from build123d import *

# Parameters (mm, degrees)
SKETCH1_W           = 5
SKETCH1_H           = 157
BOSS_EXTRUDE1_DEPTH = 30.4
SKETCH2_W           = 5
SKETCH2_H           = 2.9
BOSS_EXTRUDE2_DEPTH = 6
SKETCH3_R           = 1.05
CUT_EXTRUDE1_DEPTH  = 161.02862244
SKETCH4_R           = 2
CUT_EXTRUDE2_DEPTH  = 1.4
FILLET1_R           = 4
FILLET2_R           = 2.5


with BuildPart() as part:
    # Sketch1 → Boss-Extrude1 (new body)
    with BuildSketch(Plane(origin=(0, 0, 0), x_dir=(1, 0, 0), z_dir=(0, 1, 0))):
        with Locations((-2.5, 78.5)):
            Rectangle(SKETCH1_W, SKETCH1_H)
    extrude(amount=BOSS_EXTRUDE1_DEPTH)

    # Sketch2 → Boss-Extrude2 (add)
    with BuildSketch(Plane(origin=(0, 0, 0), x_dir=(0, 0, -1), z_dir=(1, 0, 0))):
        with Locations((2.5, 28.95)):
            Rectangle(SKETCH2_W, SKETCH2_H)
        with Locations((41.5, 28.95)):
            Rectangle(SKETCH2_W, SKETCH2_H)
        with Locations((41.5, 1.45)):
            Rectangle(SKETCH2_W, SKETCH2_H)
        with Locations((2.5, 1.45)):
            Rectangle(SKETCH2_W, SKETCH2_H)
    extrude(amount=BOSS_EXTRUDE2_DEPTH)

    # Sketch3 → Cut-Extrude1 (cut, through all)
    with BuildSketch(Plane(origin=(0, 30.4, 0), x_dir=(1, 0, 0), z_dir=(0, 1, 0))):
        with Locations(Location((3.5, 41.5, 0), (0, 0, 270))):
            Circle(SKETCH3_R)
        with Locations(Location((3.5, 2.5, 0), (0, 0, 270))):
            Circle(SKETCH3_R)
    extrude(amount=-CUT_EXTRUDE1_DEPTH, mode=Mode.SUBTRACT)

    # Sketch4 → Cut-Extrude2 (cut)
    with BuildSketch(Plane(origin=(0, 30.4, 0), x_dir=(1, 0, 0), z_dir=(0, 1, 0))):
        with Locations(Location((3.5, 41.5, 0), (0, 0, 270))):
            Circle(SKETCH4_R)
        with Locations(Location((3.5, 2.5, 0), (0, 0, 270))):
            Circle(SKETCH4_R)
    cut_extrude2 = extrude(amount=-CUT_EXTRUDE2_DEPTH, mode=Mode.SUBTRACT)

    # Mirror2: Cut-Extrude2 across plane
    add(cut_extrude2.mirror(Plane.ZX.offset(15.2)), mode=Mode.SUBTRACT)

    # Fillet1
    fillet1_edges = [part.edges().sort_by_distance(p)[0] for p in [
        (-2.5, 0, -157),
        (-5, 15.2, 0),
        (-2.5, 30.4, -157),
    ]]
    fillet(fillet1_edges, radius=FILLET1_R)

    # Fillet2
    fillet2_edges = [part.edges().sort_by_distance(p)[0] for p in [
        (6, 1.45, -5),
        (6, 1.45, 0),
        (6, 1.45, -44),
        (6, 1.45, -39),
        (6, 28.95, -44),
        (6, 28.95, -39),
        (6, 28.95, -5),
        (6, 28.95, 0),
    ]]
    fillet(fillet2_edges, radius=FILLET2_R - 0.0001)  # a hair under: the kernel refuses the full size


solid = part.part
The listing builds one solid part. Answer for the finished solid, in the listing's coordinates (mm). A direction names the side the tool comes from. Give positions to 0.01 mm unless a question says otherwise; leave off trailing zeros. Write each loop counter-clockwise with the first axis right and the second up, starting at its lowest first coordinate (ties: lowest second). Pieces come first, ordered by that corner, then holes.
Item 1: Section B-B, the plane z = -104 is taken. Write down the section's boundary in (x, y).
Item 2: Flat-ended cylindrical pins translate along their axes: P1, Ø1.2, axis at x = 3.5, z = -2, coming from the -Y side; P2, Ø5.5, axis at x = 3.5, z = -40.5, coming from the -Y side; P3, Ø3.5, axis at x = 3.5, z = -41.5, coming from the +Y side; P4, Ø1.3, axis at x = 3.5, z = -2.5, coming from the +Y side. Find the tip coordinate at first contact, or state that the pin passes through.
Item 3: Determine the mould class of faces 1 (the flat face through (2, 2.9, -41)), 2 (the cylindrical face through (5.248, 1.47, -0.713)), 3 (the flat face through (2.6, 29, -40.6)) for opening direction Y: released by +Y, released by -Y, zero draft, split by the parting line, or undercut.
Item 4: Which of the six approach directions +Z, -Z, +X, -X, +Y, -Y give full straight-line access (tool end or side, diameter ignored) to faces 4 (the flat face through (2.6, 1.4, -40.6)), 5 (the flat face through (2, 2.9, -2)), 6 (the flat face through (2, 1, -39))?
Item 5: Section A-A, the plane y = 20.5 is taken. Write down the section's boundary in (x, z), plus the area to 3 significant figures.
Item 6: Find the intervals of material crossed by line 1 along X through (y, z) = (11.5, -78.5); line 2 along X through (y, z) = (2, -2); line 3 along X through (y, z) = (29.5, -2.5), in increasing order.
Completed:
1. outline: (-5, 0) - (0, 0) - (0, 30.4) - (-5, 30.4) - close
2. P1: stops at y = 1.4
2. P2: stops at y = 0
2. P3: stops at y = 29
2. P4: passes through
3. face 1: undercut
3. face 2: zero draft
3. face 3: released by +Y
4. face 4: -Y
4. face 5: +Z, -Z, +X
4. face 6: +X, +Y, -Y
5. outline: (-5, -157) - (0, -157) - (0, 0) - (-1, 0) arc R4 ccw to (-5, -4) - close
5. area: 782 mm2
6. line 1: x = -5 to 0
6. line 2: x = -4.46 to 2.58, 4.42 to 5.95
6. line 3: x = -4.71 to 1.5, 5.5 to 6
